Read the model definition and answer for the solid it produces. Units are mm, in the model's axes. Face numbers are marked on the shaded views. Coordinates: 2 decimals unless noted, no trailing zeros. Write each loop counter-clockwise with the first axis right and the second up, starting at its lowest first coordinate (ties: lowest second). Pieces come first, ordered by that corner, then holes. Notation, with made-up numbers: (-9, 55) -> (29, 55) arc R30 cw to (29, 81) -> close; hole circle Ø3 at (-30.5, 52.25). An arc over 180 degrees is marked (long way). One line per item, written item: value. Start each with the question number.
1. Find section A-A, the plane y = 0. Write down the section's boundary in (x, z), and give its area (3 significant figures).
2. Find section B-B, the plane x = 12. Write down the section's boundary in (y, z).
3. Find section D-D, the plane z = 4.35. Write down the section's boundary in (x, y), and give its area (3 significant figures).
4. Given P1, Ø1.5, axis at x = -6.5, y = 2.5, coming from the -Z side; P2, Ø9.5, axis at x = 0, y = 0, coming from the -Z side, each flat-ended and moving along its own axis, determine where each tip first touches the part or whether it passes through.
5. For a pull along Y with two mould halves and no side action, classify the marked faces 1, 2, 3 and 4 as pulls with the +Y half, pulls with the -Y half, needs draft (parallel to the pull), parting line crosses it, or undercut.
6. Consider line 1 along X through (y, z) = (-1.75, 3.65); line 2 along Y through (x, z) = (-4, 2.4); line 3 along X through (y, z) = (2, 0.6). Determine where each line is inside the solid, lowest interval first.
7. Find section C-C, the plane y = -5.5. Write down the section's boundary in (x, z).
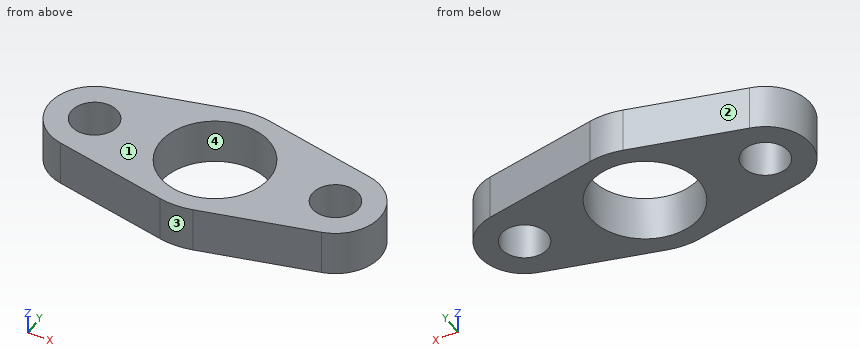
Autodesk Fusion 360 part; units mm, degrees
sketch "Sketch1" plane through (0, 0, 0) normal (0, 0, 1) x (1, 0, 0)
  circle A0 centre (-13.3, 0) radius 2.55
  circle A1 centre (-13.3, 0) radius 5
  line L0 (0, 10) -> (0, 0) construction
  circle A2 centre (13.3, 0) radius 2.55
  circle A3 centre (13.3, 0) radius 5
  circle A4 centre (0, 0) radius 6
  circle A5 centre (0, 0) radius 8
  line L1 (-14.2326, 4.9123) -> (-1.8069, 7.7933)
  line L2 (1.8045, 7.7938) -> (14.4278, 4.8711)
  line L3 (1.8045, -7.7938) -> (14.4278, -4.8711)
  line L4 (-14.4278, -4.8711) -> (-1.8045, -7.7938)
  circle A6 centre (-13.3, 0) radius 1.5
  circle A7 centre (13.3, 0) radius 1.5
  dimension "d1" = 5.1
  dimension "d2" = 13.3
  dimension "d3" = 10
  dimension "d6" = 12
  dimension "d7" = 16
  dimension "d10" = 3
extrude "Extrude2" add sketch "Sketch1" along normal blind 5 contours A1 | A1 A5 L1 L4 | A5 | A3 A5 L2 L3 | A3
equation "d2 = ( 26.6 / 2 ) * 1 mm"
Answer block:
1. outline: (-18.3, 0) -> (-15.85, 0) -> (-15.85, 5) -> (-18.3, 5) -> close; (-10.75, 0) -> (-6, 0) -> (-6, 5) -> (-10.75, 5) -> close; (6, 0) -> (10.75, 0) -> (10.75, 5) -> (6, 5) -> close; (15.85, 0) -> (18.3, 0) -> (18.3, 5) -> (15.85, 5) -> close
1. area: 72.0 mm2
2. outline: (-5.43, 0) -> (-2.19, 0) -> (-2.19, 5) -> (-5.43, 5) -> close; (2.19, 0) -> (5.43, 0) -> (5.43, 5) -> (2.19, 5) -> close
3. outline: (-14.43, -4.87) -> (-1.8, -7.79) arc R8 ccw to (1.8, -7.79) -> (14.43, -4.87) arc R5 ccw to (14.43, 4.87) -> (1.8, 7.79) arc R8 ccw to (-1.81, 7.79) -> (-14.23, 4.91) arc R5 ccw to start; hole circle Ø5.1 at (-13.3, 0); hole circle Ø12 at (0, 0); hole circle Ø5.1 at (13.3, 0)
3. area: 279 mm2
4. P1: stops at z = 0
4. P2: passes through
5. face 1: needs draft
5. face 2: pulls with the +Y half
5. face 3: pulls with the -Y half
5. face 4: undercut
6. line 1: x = -17.98 to -15.15, -11.45 to -5.74, 5.74 to 11.45, 15.15 to 17.98
6. line 2: y = -7.29 to -4.47, 4.47 to 7.28
6. line 3: x = -17.88 to -14.88, -11.72 to -5.66, 5.66 to 11.72, 14.88 to 17.88
7. outline: (-11.71, 0) -> (-2.4, 0) -> (-2.4, 5) -> (-11.71, 5) -> close; (2.4, 0) -> (11.71, 0) -> (11.71, 5) -> (2.4, 5) -> close
